```python
from build123d import *

# Parameters (mm, degrees)
SKETCH1_R           = 15
SKETCH1_R_2         = 12
SKETCH1_R_3         = 1
BOSS_EXTRUDE1_DEPTH = 1
SKETCH2_R           = 15
SKETCH2_R_2         = 12
SKETCH2_R_3         = 1
BOSS_EXTRUDE3_DEPTH = 1.5


with BuildPart() as part:
    # Sketch1 → Boss-Extrude1 (new body)
    with BuildSketch(Plane.XY):
        Circle(SKETCH1_R)
        Circle(SKETCH1_R_2, mode=Mode.SUBTRACT)
        with Locations((0, 13.5)):
            Circle(SKETCH1_R_3, mode=Mode.SUBTRACT)
        with Locations((13.5, 0)):
            Circle(SKETCH1_R_3, mode=Mode.SUBTRACT)
        with Locations((0, -13.5)):
            Circle(SKETCH1_R_3, mode=Mode.SUBTRACT)
        with Locations((-13.5, 0)):
            Circle(SKETCH1_R_3, mode=Mode.SUBTRACT)
    extrude(amount=BOSS_EXTRUDE1_DEPTH)

    # Sketch2 → Boss-Extrude3 (add)
    with BuildSketch(Plane.XY.offset(1)):
        Circle(SKETCH2_R)
        Circle(SKETCH2_R_2, mode=Mode.SUBTRACT)
        with Locations((0, 13.5)):
            Circle(SKETCH2_R_3, mode=Mode.SUBTRACT)
        with Locations((13.5, 0)):
            Circle(SKETCH2_R_3, mode=Mode.SUBTRACT)
        with Locations((0, -13.5)):
            Circle(SKETCH2_R_3, mode=Mode.SUBTRACT)
        with Locations((-13.5, 0)):
            Circle(SKETCH2_R_3, mode=Mode.SUBTRACT)
    extrude(amount=BOSS_EXTRUDE3_DEPTH)


solid = part.part
```
CAD build for the part. Positions are in the model's coordinates, mm. Coordinates: 2 decimals unless noted, no trailing zeros. Loops run counter-clockwise (first coordinate to the right, second up) from the corner with the lowest first, then second, coordinate; pieces in that order, holes last. Notation, with made-up numbers: (87, 40.25) - (145, 40.25) arc R28 cw to (145, 62.25) - close; hole circle Ø1 at (40, 15). An arc over 180 degrees is marked (long way). Return JSON: item names as keys, results as strings.
1. Drop flat-ended pins along their axis: pin 1 (1.8 mm diameter, centred on x = -13.5, y = 0, fed in from -Z); pin 2 (2.5 mm diameter, centred on x = 0, y = -13.5, fed in from +Z); pin 3 (1 mm diameter, centred on x = 4, z = 0.5, fed in from +Y). Give the stop position or say it passes through.
Result:
{"pin 1": "passes through", "pin 2": "stops at z = 2.5", "pin 3": "stops at y = 14.59"}
2. Probe L1, parallel to Y at x = 0, z = 1.7; L2, parallel to Y at x = 2.5, z = 1.2; L3, parallel to X at y = -11, z = 0.55. List the from-to ranges inside material, lowest first. Write a range as from..to.
Result:
{"L1": "y = -15..-14.5, -12.5..-12, 12..12.5, 14.5..15", "L2": "y = -14.79..-11.74, 11.74..14.79", "L3": "x = -10.2..-4.8, 4.8..10.2"}
3. Band-saw the part on C-C (z = 1.05). Give the cut face in (x, y), and give its area (3 significant figures).
Result:
{"outline": "circle Ø30 at (0, 0); hole circle Ø2 at (-13.5, 0); hole circle Ø24 at (0, 0); hole circle Ø2 at (0, -13.5); hole circle Ø2 at (0, 13.5); hole circle Ø2 at (13.5, 0)", "area": "242 mm2"}
4. Mould opens along X. For faces 1 (the cylindrical face through (-14.985, 0.66, 1.232)), 2 (the flat face through (-10, 7, 0)), 3 (the cylindrical face through (-12.546, 0.3, 1.232)) say: released by +X, released by -X, zero draft, split by the parting line, or undercut.
Result:
{"face 1": "split by the parting line", "face 2": "zero draft", "face 3": "undercut"}
5. Band-saw the part on A-A (y = 0). Give the cut face in (x, z), and give its area (3 significant figures).
Result:
{"outline": "(-15, 0) - (-14.5, 0) - (-14.5, 2.5) - (-15, 2.5) - close; (-12.5, 0) - (-12, 0) - (-12, 2.5) - (-12.5, 2.5) - close; (12, 0) - (12.5, 0) - (12.5, 2.5) - (12, 2.5) - close; (14.5, 0) - (15, 0) - (15, 2.5) - (14.5, 2.5) - close", "area": "5.00 mm2"}
6. Band-saw the part on D-D (x = 7.75). Give the cut face in (y, z).
Result:
{"outline": "(-12.84, 0) - (-9.16, 0) - (-9.16, 2.5) - (-12.84, 2.5) - close; (9.16, 0) - (12.84, 0) - (12.84, 2.5) - (9.16, 2.5) - close"}
